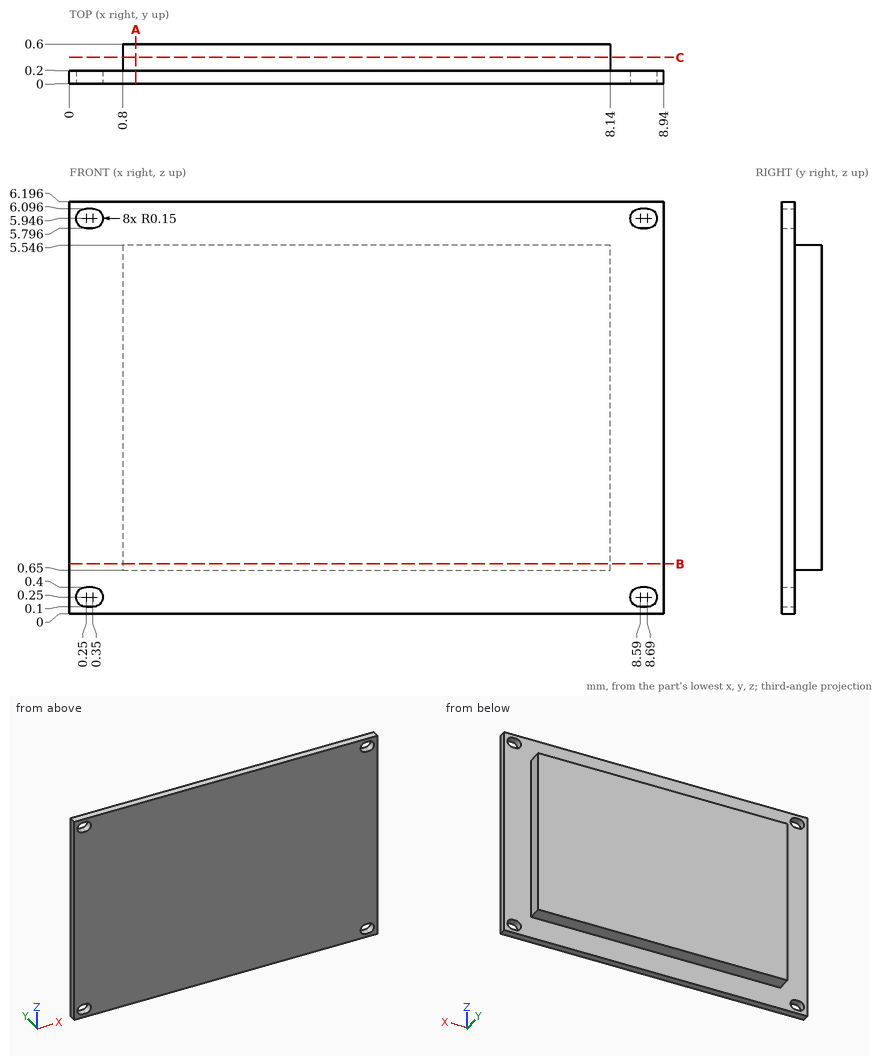
Could you check a few things on this drawing? It's one solid part, dimensions in mm from its lowest x, y, z. Coordinates: 2 decimals unless noted, no trailing zeros. Write each loop counter-clockwise with the first axis right and the second up, starting at its lowest first coordinate (ties: lowest second). Pieces come first, ordered by that corner, then holes. Notation, with made-up numbers: M -25,77 L 24,77 A35 ccw 24,112 Z; hole C 29.25,89 d4. An arc over 180 degrees is marked long. One line per question, with ' | ' between items.
1) Imagine slicing it at C-C, the plane y = 0.4. Write out the boundary of the cut face in (x, z).
Checks:
outline: M 0.8,0.65 L 8.14,0.65 L 8.14,5.55 L 0.8,5.55 Z
2) Imagine slicing it at B-B, the plane z = 0.75. Write out the boundary of the cut face in (x, y), and give its area (3 significant figures).
Checks:
outline: M 0,0 L 8.94,0 L 8.94,0.2 L 8.14,0.2 L 8.14,0.6 L 0.8,0.6 L 0.8,0.2 L 0,0.2 Z | area: 4.72 mm²
3) Imagine slicing it at A-A, the plane x = 1. Write out the boundary of the cut face in (y, z), and give its area (3 significant figures).
Checks:
outline: M 0,0 L 0.2,0 L 0.2,0.65 L 0.6,0.65 L 0.6,5.55 L 0.2,5.55 L 0.2,6.2 L 0,6.2 Z | area: 3.20 mm²
4) I need wall thicknesses on probe 1 along X at (y, z) = (0.55, 4); probe 2 along Z at (x, y) = (1.5, 0.3); probe 3 along Y at (x, z) = (3.5, 6). Which ranges of each line are inside material? Lowest first, please. Write a range as [from, to].
Checks:
probe 1: [0.8, 8.14] | probe 2: [0.65, 5.55] | probe 3: [0, 0.2]
